Autodesk Inventor part; units mm, degrees
ref_plane "Work Plane1" through (-20.8033, -6.3, -5.9) normal (0, 0, 1) x (1, 0, 0)
ref_plane "YZ Plane" through (0, 0, 0) normal (1, 0, 0) x (0, 1, 0)
ref_plane "XZ Plane" through (0, 0, 0) normal (0, 1, 0) x (-1, 0, 0)
sketch "Sketch1" plane through (0, 0, 0) normal (0, 0, 1) x (1, 0, 0)
  line L0 (0.8467, -0.7217) -> (0.8467, 0.7217) construction
  line L1 (0.8467, 0.7217) -> (2.0967, 1.4434) construction
  line L2 (2.0967, 1.4434) -> (3.3467, 0.7217) construction
  line L3 (3.3467, 0.7217) -> (3.3467, -0.7217) construction
  line L4 (3.3467, -0.7217) -> (2.0967, -1.4434) construction
  line L5 (2.0967, -1.4434) -> (0.8467, -0.7217) construction
  circle A0 centre (2.0967, 0) radius 2.45 construction
  line L6 (4.8467, -1.5877) -> (3.4717, -2.3816) construction
  line L7 (15.0967, 3) -> (15.0967, -3) construction
  line L8 (-10.9033, 3) -> (-10.9033, -3) construction
  line L9 (-0.6533, 0) -> (-0.6533, 1.5877) construction
  circle A1 centre (2.0967, 0) radius 5
  circle A2 centre (2.0967, 0) radius 1.7
  line L10 (-10.9033, -3) -> (15.0967, -3)
  line L11 (-10.9033, 3) -> (15.0967, 3)
  circle A3 centre (2.0967, 0) radius 3.5
  circle A4 centre (2.0967, 0) radius 6.5
  point P0 (0.4719, -0.5)
  point P1 (3.7215, -0.5)
  dimension "d10" = 7
  dimension "d13" = 13
ref_plane "Work Plane1" through (-20.8033, -6.3, -5.9) normal (0, 0, 1) x (1, 0, 0)
extrude "Extrusion1" add sketch "Sketch1" against normal blind 4 contours A1 L10 A3 L11 | A1 L11 A4 L10 | L11 A3 A1 | A1 L11 A4 | L10 A4 A1 | A1 L10 A3 | L11 A3 L10 A1 | A1 L10 A4 L11
sketch "Sketch2" plane through (2.0967, 0, 0) normal (0, 0, 1) x (1, 0, 0)
  line L0 (-2, 1.5) -> (2, 1.5) construction
  arc A0 (2.5, 0) -> (2, 1.5) centre (0, 0) ccw construction
  arc A1 (-2, 1.5) -> (-2.5, 0) centre (0, 0) ccw construction
  line L1 (2, -1.5) -> (-2, -1.5) construction
  arc A2 (-2.5, 0) -> (2.5, 0) centre (0, 0) ccw construction
  line L2 (2.0248, 1.55) -> (-2.0248, 1.55) construction
  arc A3 (-2.0248, 1.55) -> (-2.55, 0) centre (0, 0) ccw construction
  arc A4 (-2.55, 0) -> (2.55, 0) centre (0, 0) ccw construction
  arc A5 (2.55, 0) -> (2.0248, 1.55) centre (0, 0) ccw construction
  line L3 (-2.0248, 1.55) -> (2.0248, 1.55) construction
  line L4 (-2.0248, 1.55) -> (2.0248, 1.55)
  line L5 (-2.0248, -1.55) -> (2.0248, -1.55)
  arc A6 (-2.0248, 1.55) -> (-2.0248, -1.55) centre (0, 0) ccw
  arc A7 (2.0248, -1.55) -> (2.0248, 1.55) centre (0, 0) ccw
  circle A8 centre (0, 0) radius 6.5
  point P0 (-2.0967, 0)
  dimension "d11" = 3.1
  dimension "d12" = 2.55
extrude "Extrusion2" add sketch "Sketch2" along normal blind 5
chamfer "Chamfer1" distance 1.2 angle 45 4 edges at (2.0967, 1.55, 5) (-0.4533, 0, 5) (2.0967, -1.55, 5) (4.6467, 0, 5)
sketch "Sketch3" plane through (0, 0, 0) normal (0, 1, 0) x (-1, 0, 0)
  line L0 (-4.6467, 0) -> (-4.6467, 3.8)
  line L1 (0.4533, 0) -> (0.4533, 3.8)
  line L2 (-8.5967, -4) -> (4.4033, -4)
  circle A0 centre (-2.0967, -1.5) radius 1.25
  line L3 (-8.5967, -4) -> (4.4033, -4)
  point P0 (0, 0)
  point P1 (-8.5967, 0)
  point P2 (4.4033, 0)
  dimension "d14" = 2.5
  dimension "d15" = 2.5
extrude "Extrusion3" cut sketch "Sketch3" against normal blind 10
pattern_circular "Circular Pattern1" count 3 over 360 about axis through (2.0967, 0, 0) along (0, 0, -1) of "Extrusion3"
sketch "Sketch4" plane through (0.0718, -1.55, 0) normal (0, 1, 0) x (1, 0, 0)
  line L0 (0, -3.8) -> (4.0497, -3.8)
  line L1 (-4.4752, -5) -> (8.5248, -5)
  line L2 (8.5248, 4) -> (-4.4752, 4)
  line L3 (4.0497, -3.8) -> (0, -3.8)
  line L4 (4.0497, 0) -> (4.0497, -3.8)
  line L5 (0, 0) -> (4.0497, 0)
  line L6 (0, 0) -> (0, -3.8)
  circle A0 centre (2.0248, -2.0248) radius 2.0248
  point P0 (-0.0718, 0)
  point P1 (8.1739, 1.5)
  point P2 (-2.8742, 1.5)
  point P3 (0.7748, 1.5)
hole "Hole1" at (2.0967, -1.55, 2.0248) direction (0, -1, 0) diameter 2.5 end through all both
properties part number "01_28BYJ_Coupling_ScrewM4"
Check sheet for the modelled part. Datum: model origin and axes. Units: mm. A direction names the side the tool comes from. Give positions to 0.01 mm unless a question says otherwise; leave off trailing zeros. Order: outer loops, then holes, each group sorted by start corner. A loop starts at its lowest first (then second) coordinate and runs counter-clockwise, first axis right, second up. Notation, with made-up numbers: (14.5, 33.5) -> (60.5, 33.5) arc R22 ccw to (60.5, 65.5) -> close; hole circle Ø4 at (59, -7). An arc over 180 degrees is marked (long way). Use CSV: the item, a comma, the result in double quotes. Start each with the question number.
1) Sectioned sample at D-D, the plane x = 2.75. Record the boundary of the cut face in (y, z), plus the area to 3 significant figures.
2) Sectioned sample at A-A, the plane y = 0. Record the boundary of the cut face in (x, z).
3) Go/stop test with flat-tipped pins: P1, Ø1, axis at y = 5, z = -0.5, coming from the -X side; P2, Ø2, axis at y = 1.5, z = -2, coming from the -X side; P3, Ø3.5, axis at x = 1, y = 0.5, coming from the -Z side; P4, Ø3, axis at x = 1.5, z = 2.5, coming from the +Y side. Record where each tip stops, or that it passes through.
4) Sectioned sample at B-B, the plane z = -1.5. Record the boundary of the cut face in (x, y).
5) Material ranges on line 1 (Z direction, x = 2.25, y = -5.25); line 2 (X direction, y = 0, z = -1.75); line 3 (Z direction, x = -1.5, y = 2), recorded low to high. Write a range as from..to.
6) Mould release check, pull along Z, two halves, no side actions. Record for faces 1 (the face through (5.68, 3.51, -1.45)), 2 (the face through (2.06, 2.14, 4.39)), 3 (the face through (4.647, 0.023, 1.873)): released by +Z, released by -Z, zero draft, split by the parting line, or undercut.
7) Set-up check for faces 4 (the face through (-1.4, 0.15, -1.97)), 5 (the face through (3.345, -4.862, -1.445)), 6 (the face through (2.1, 1.55, 0.6)): record each of +Z, -Z, +X, -X, +Y, -Y from which the full face is reachable in a straight line by a thin tool's end or side.
8) Sectioned sample at C-C, the plane z = 0.25. Record the boundary of the cut face in (x, y).
Recorded:
1,outline,"(-6.47, -4) -> (-3.44, -4) -> (-3.44, -2.57) -> (-6.47, -2.57) -> close; (-6.47, -0.43) -> (-3.44, -0.43) -> (-3.44, 0) -> (-1.55, 0) -> (-1.55, 0.96) -> (-6.47, 0.96) -> close; (-6.47, 3.09) -> (-1.55, 3.09) -> (-1.55, 3.8) -> (-2.75, 5) -> (-6.47, 5) -> close; (1.55, 0) -> (3.44, 0) -> (3.44, -4) -> (6.47, -4) -> (6.47, 0.96) -> (1.55, 0.96) -> close; (1.55, 3.09) -> (6.47, 3.09) -> (6.47, 5) -> (2.75, 5) -> (1.55, 3.8) -> close"
1,area,"44.5 mm2"
2,outline,"(-4.4, -4) -> (-1.4, -4) -> (-1.4, 0) -> (-0.45, 0) -> (-0.45, 3.8) -> (-1.65, 5) -> (-4.4, 5) -> close; (4.65, 0) -> (5.6, 0) -> (5.6, -4) -> (8.6, -4) -> (8.6, 5) -> (5.85, 5) -> (4.65, 3.8) -> close"
3,P1,"x = -2.59"
3,P2,"x = -4.38"
3,P3,"z = 0"
3,P4,"y = 6.5"
4,outline,"(-4.05, 2.11) arc R6.5 ccw to (0.85, -6.38) -> (0.85, -3.27) arc R3.5 cw to (-1.36, 0.55) -> close; (-2.8, 4.27) -> (-0.11, 2.72) arc R3.5 cw to (4.3, 2.72) -> (7, 4.27) arc R6.5 ccw to start; (3.35, -6.38) arc R6.5 ccw to (8.25, 2.11) -> (5.55, 0.55) arc R3.5 cw to (3.35, -3.27) -> close"
5,line 1,"-4..-2.74, -0.26..0.78, 3.27..5"
5,line 2,"-4.4..-1.4, 5.6..8.6"
5,line 3,"-4..-2.75, -0.25..5"
6,face 1,"undercut"
6,face 2,"released by +Z"
6,face 3,"zero draft"
7,face 4,"-Z"
7,face 5,"-Y"
7,face 6,"+Z, -Z"
8,outline,"circle Ø13 at (2.1, 0); hole (0.07, -1.55) -> (4.12, -1.55) arc R2.55 ccw to (4.12, 1.55) -> (0.07, 1.55) arc R2.55 ccw to start"
